Design review of the part built by this model. Coordinates are the model's own, in mm. Coordinates: 2 decimals unless noted, no trailing zeros. Write each loop counter-clockwise with the first axis right and the second up, starting at its lowest first coordinate (ties: lowest second). Pieces come first, ordered by that corner, then holes.
Q1. Add section C-C, the plane z = -6. Give the boundary of the cut face in (x, y), plus the area to 3 significant figures.
Q2. Add section B-B, the plane y = 47. Give the boundary of the cut face in (x, z).
Q3. Add section A-A, the plane x = 43.5. Give the boundary of the cut face in (y, z), plus the area to 3 significant figures.
Q4. To check wall thickness, follow probe 1 along X at (y, z) = (47.9, -26); probe 2 along Z at (x, y) = (43.5, 46.4); probe 3 along X at (y, z) = (49.7, -25). State the ranges of each line that lie inside material, in increasing order.
from build123d import *

# Parameters (mm, degrees)
SKETCH1_W           = 55
SKETCH1_H           = 32
BOSS_EXTRUDE1_DEPTH = 50
SKETCH2_W           = 45
SKETCH2_H           = 32
CUT_EXTRUDE1_DEPTH  = 45
SKETCH3_R           = 1.75
CUT_EXTRUDE2_DEPTH  = 51
SKETCH4_R           = 1.75
CUT_EXTRUDE3_DEPTH  = 56
SKETCH5_W           = 1.1
SKETCH5_H           = 35
CUT_EXTRUDE4_DEPTH  = 1.2
SKETCH6_W           = 5
SKETCH6_H           = 32
CUT_EXTRUDE5_DEPTH  = 51


with BuildPart() as part:
    # Sketch1 → Boss-Extrude1 (new body)
    with BuildSketch(Plane(origin=(0, 0, 0), x_dir=(1, 0, 0), z_dir=(0, 1, 0))):
        with Locations((27.5, 16)):
            Rectangle(SKETCH1_W, SKETCH1_H)
    extrude(amount=BOSS_EXTRUDE1_DEPTH)

    # Sketch2 → Cut-Extrude1 (cut)
    with BuildSketch(Plane.XZ):
        with Locations((27.5, -16)):
            Rectangle(SKETCH2_W, SKETCH2_H)
    extrude(amount=-CUT_EXTRUDE1_DEPTH, mode=Mode.SUBTRACT)

    # Sketch3 → Cut-Extrude2 (cut, through all)
    with BuildSketch(Plane(origin=(0, 50, 0), x_dir=(1, 0, 0), z_dir=(0, 1, 0))):
        with Locations((43.5, 26)):
            Circle(SKETCH3_R)
        with Locations((43.5, 6)):
            Circle(SKETCH3_R)
        with Locations((11.5, 26)):
            Circle(SKETCH3_R)
        with Locations((11.5, 6)):
            Circle(SKETCH3_R)
    extrude(amount=-CUT_EXTRUDE2_DEPTH, mode=Mode.SUBTRACT)

    # Sketch4 → Cut-Extrude3 (cut, through all)
    with BuildSketch(Plane(origin=(55, 0, 0), x_dir=(0, 0, -1), z_dir=(1, 0, 0))):
        with Locations((6, 5)):
            Circle(SKETCH4_R)
        with Locations((26, 5)):
            Circle(SKETCH4_R)
    extrude(amount=-CUT_EXTRUDE3_DEPTH, mode=Mode.SUBTRACT)

    # Sketch5 → Cut-Extrude4 (cut)
    with BuildSketch(Plane.ZY.offset(-50)):
        with Locations((-29.45, 27.5)):
            Rectangle(SKETCH5_W, SKETCH5_H)
        with Locations((-31.45, 27.5)):
            Rectangle(SKETCH5_W, SKETCH5_H)
        with Locations((-27.45, 27.5)):
            Rectangle(SKETCH5_W, SKETCH5_H)
        with Locations((-25.45, 27.5)):
            Rectangle(SKETCH5_W, SKETCH5_H)
        with Locations((-23.45, 27.5)):
            Rectangle(SKETCH5_W, SKETCH5_H)
        with Locations((-21.45, 27.5)):
            Rectangle(SKETCH5_W, SKETCH5_H)
        with Locations((-19.45, 27.5)):
            Rectangle(SKETCH5_W, SKETCH5_H)
        with Locations((-17.45, 27.5)):
            Rectangle(SKETCH5_W, SKETCH5_H)
        with Locations((-15.45, 27.5)):
            Rectangle(SKETCH5_W, SKETCH5_H)
        with Locations((-13.45, 27.5)):
            Rectangle(SKETCH5_W, SKETCH5_H)
        with Locations((-11.45, 27.5)):
            Rectangle(SKETCH5_W, SKETCH5_H)
        with Locations((-9.45, 27.5)):
            Rectangle(SKETCH5_W, SKETCH5_H)
        with Locations((-7.45, 27.5)):
            Rectangle(SKETCH5_W, SKETCH5_H)
        with Locations((-5.45, 27.5)):
            Rectangle(SKETCH5_W, SKETCH5_H)
        with Locations((-3.45, 27.5)):
            Rectangle(SKETCH5_W, SKETCH5_H)
        with Locations((-1.45, 27.5)):
            Rectangle(SKETCH5_W, SKETCH5_H)
        with Locations((0.55, 27.5)):
            Rectangle(SKETCH5_W, SKETCH5_H)
    extrude(amount=-CUT_EXTRUDE4_DEPTH, mode=Mode.SUBTRACT)

    # Sketch6 → Cut-Extrude5 (cut, through all)
    with BuildSketch(Plane(origin=(0, 50, 0), x_dir=(1, 0, 0), z_dir=(0, 1, 0))):
        with Locations((52.5, 16)):
            Rectangle(SKETCH6_W, SKETCH6_H)
        with Locations((2.5, 16)):
            Rectangle(SKETCH6_W, SKETCH6_H)
    extrude(amount=-CUT_EXTRUDE5_DEPTH, mode=Mode.SUBTRACT)


solid = part.part
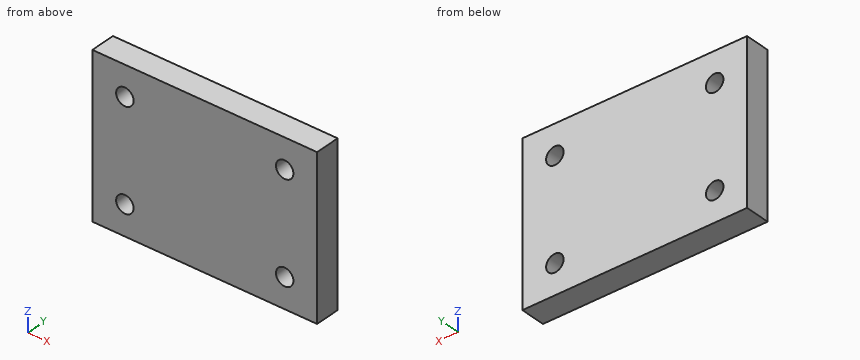
Here are the results:
1. outline: (5, 45) - (9.75, 45) - (9.75, 50) - (5, 50) - close; (13.25, 45) - (41.75, 45) - (41.75, 50) - (13.25, 50) - close; (45.25, 45) - (50, 45) - (50, 50) - (45.25, 50) - close
1. area: 190 mm2
2. outline: (5, -32) - (50, -32) - (50, 0) - (5, 0) - close; hole circle Ø3.5 at (11.5, -26); hole circle Ø3.5 at (11.5, -6); hole circle Ø3.5 at (43.5, -26); hole circle Ø3.5 at (43.5, -6)
3. outline: (45, -32) - (50, -32) - (50, -27.75) - (45, -27.75) - close; (45, -24.25) - (50, -24.25) - (50, -7.75) - (45, -7.75) - close; (45, -4.25) - (50, -4.25) - (50, 0) - (45, 0) - close
3. area: 125 mm2
4. probe 1: x = 5 to 9.75, 13.25 to 41.75, 45.25 to 50
4. probe 2: z = -32 to -27.75, -24.25 to -7.75, -4.25 to 0
4. probe 3: x = 5 to 10.06, 12.94 to 42.06, 44.94 to 50
